Can you work these out from the model? Positions are in its coordinate system, mm. A direction names the side the tool comes from. Round coordinates to 2 decimals unless told otherwise and drop trailing zeros. Loops run counter-clockwise (first coordinate to the right, second up) from the corner with the lowest first, then second, coordinate; pieces in that order, holes last. Notation, with made-up numbers: (26, 43) -> (67, 43) arc R13 ccw to (67, 57) -> close; hole circle Ø5 at (13, 29.5). An arc over 180 degrees is marked (long way). Use a Markdown table: item, result.
from build123d import *

# Parameters (mm, degrees)
F0_R     = 22.225
F1_DEPTH = 76.2
F2_R     = 12.7
F4_DEPTH = 56.642
F3_R     = 15.875
F5_DEPTH = 101.6


with BuildPart() as f1:
    # F0 (on Front) → F1 (new body)
    with BuildSketch(Plane.XZ):
        with BuildLine():
            Line((-149.225, 0), (0, 0))
            Line((0, 0), (0, 50.8))
            Line((0, 50.8), (-76.2, 50.8))
            Line((-76.2, 50.8), (-76.2, 101.6))
            Line((-76.2, 101.6), (0, 101.6))
            Line((0, 101.6), (0, 152.4))
            Line((0, 152.4), (-149.225, 152.4))
            ThreePointArc((-149.225, 152.4), (-225.425, 76.2), (-149.225, 0))
        make_face()
        with Locations((-114.3, 76.2)):
            Circle(F0_R, mode=Mode.SUBTRACT)
    extrude(amount=F1_DEPTH)

    # F2 (on face) → F4 (cut)
    with BuildSketch(Plane.XY.offset(152.4)):
        with Locations((-38.1, -38.1)):
            Circle(F2_R)
    extrude(amount=-F4_DEPTH, mode=Mode.SUBTRACT)

    # F3 (on face) → F5 (cut)
    with BuildSketch(Plane.XY.offset(50.8)):
        with Locations((-38.1, -38.1)):
            Circle(F3_R)
    extrude(amount=-F5_DEPTH, mode=Mode.SUBTRACT)


solid = f1.part
1. Which directions (+Z, -Z, +X, -X, +Y, -Y) give clear straight access to the entire face, cutting with the end or side of a thin tool? Please do faces 4 (the cylindrical face through (-23.436, -44.18, 25.756)), 5 (the flat face through (-54.5, -37.6, 50.8)), 6 (the flat face through (0, -38, 25)).
Answer sheet:
| item | result |
|---|---|
| face 4 | -Z |
| face 5 | +X, +Y, -Y |
| face 6 | +Z, -Z, +X, +Y, -Y |
2. I need wall thicknesses on line 1 (Y direction, x = -38.1, z = 19) (3 decimals); line 2 (Z direction, x = -11.5, y = -4); line 3 (Z direction, x = -114.3, y = -16) (3 decimals). Which ranges of each line are inside material? Lowest first, please.
Answer sheet:
| item | result |
|---|---|
| line 1 | y = -76.2 to -53.975, -22.225 to 0 |
| line 2 | z = 0 to 50.8, 101.6 to 152.4 |
| line 3 | z = 0 to 53.975, 98.425 to 152.4 |
3. I want a section at D-D (x = -119). Please give me the cut outline in (y, z), plus the area to 3 significant figures.
Answer sheet:
| item | result |
|---|---|
| outline | (-76.2, 0) -> (0, 0) -> (0, 54.48) -> (-76.2, 54.48) -> close; (-76.2, 97.92) -> (0, 97.92) -> (0, 152.4) -> (-76.2, 152.4) -> close |
| area | 8,300 mm² |
4. I want a section at B-B (x = -38.1). Please give me the cut outline in (y, z) (3 decimals).
Answer sheet:
| item | result |
|---|---|
| outline | (-76.2, 0) -> (-53.975, 0) -> (-53.975, 50.8) -> (-76.2, 50.8) -> close; (-76.2, 101.6) -> (-50.8, 101.6) -> (-50.8, 152.4) -> (-76.2, 152.4) -> close; (-25.4, 101.6) -> (0, 101.6) -> (0, 152.4) -> (-25.4, 152.4) -> close; (-22.225, 0) -> (0, 0) -> (0, 50.8) -> (-22.225, 50.8) -> close |
5. Will these pins go through, and if not, where does the flat tip stop? pin 1 Ø6 at (x, z) = (-197, 49) entering from +Y; pin 2 Ø1 at (y, z) = (-17.5, 33.5) entering from -X.
Answer sheet:
| item | result |
|---|---|
| pin 1 | stops at y = 0 |
| pin 2 | stops at x = -212.67 |
6. I want a section at A-A (y = -38.1). Please give me the cut outline in (x, z) (3 decimals).
Answer sheet:
| item | result |
|---|---|
| outline | (-149.225, 0) -> (-53.975, 0) -> (-53.975, 50.8) -> (-76.2, 50.8) -> (-76.2, 101.6) -> (-50.8, 101.6) -> (-50.8, 152.4) -> (-149.225, 152.4) arc R76.2 ccw to start; (-25.4, 101.6) -> (0, 101.6) -> (0, 152.4) -> (-25.4, 152.4) -> close; (-22.225, 0) -> (0, 0) -> (0, 50.8) -> (-22.225, 50.8) -> close; hole circle Ø44.45 at (-114.3, 76.2) |
7. I want a section at C-C (z = 76.2). Please give me the cut outline in (x, y) (3 decimals), plus the area to 3 significant figures.
Answer sheet:
| item | result |
|---|---|
| outline | (-225.425, -76.2) -> (-136.525, -76.2) -> (-136.525, 0) -> (-225.425, 0) -> close; (-92.075, -76.2) -> (-76.2, -76.2) -> (-76.2, 0) -> (-92.075, 0) -> close |
| area | 7,980 mm² |
8. If we mould it in two halves opening along X, with no side actions, what happens to faces 1 (the flat face through (-56, -38, 101.6)), 2 (the cylindrical face through (-48.2, -45.8, 127.4)), 3 (the flat face through (-76.2, -38, 76))? For each: +X half, -X half, draft (parallel to the pull), parting line (faces both ways), or undercut.
Answer sheet:
| item | result |
|---|---|
| face 1 | draft |
| face 2 | undercut |
| face 3 | +X half |
